```python
from build123d import *
from OCP.BRepFilletAPI import BRepFilletAPI_MakeChamfer

# Parameters (mm, degrees)
SKETCH1_W           = 60.325
SKETCH1_H           = 60.325
SKETCH1_R           = 1.778
SKETCH1_R_2         = 1.524
BOSS_EXTRUDE1_DEPTH = 6
CUT_EXTRUDE1_DEPTH  = 44.076128105
FILLET7_R           = 1.27
FILLET8_R           = 1.27
FILLET9_R           = 2.54
FILLET15_R          = 5.08
SKETCH4_W           = 2.54
SKETCH4_H           = 1.5875
BOSS_EXTRUDE2_DEPTH = 6
SKETCH6_W           = 12.7
SKETCH6_H           = 6.35
BOSS_EXTRUDE3_DEPTH = 6
FILLET10_R          = 2.54
FILLET11_R          = 2.54
BOSS_EXTRUDE4_DEPTH = 6
FILLET12_R          = 5.08
FILLET13_R          = 5.08
CUT_EXTRUDE2_REACH  = 52.712
SKETCH9_W           = 6.858
SKETCH9_H           = 2.9972
CHAMFER1_SIZE       = 0.381
CHAMFER1_SIZE2      = 1.046788897
FILLET14_R          = 0.508


with BuildPart() as part:
    # Sketch1 → Boss-Extrude1 (new body)
    with BuildSketch(Plane.XY):
        Rectangle(SKETCH1_W, SKETCH1_H)
        with Locations((26.289, 23.5585)):
            Circle(SKETCH1_R, mode=Mode.SUBTRACT)
        with Locations(Location((26.289, -23.5585, 0), (0, 0, 180))):
            Circle(SKETCH1_R, mode=Mode.SUBTRACT)
        with Locations((-25.4, 25.4)):
            Circle(SKETCH1_R, mode=Mode.SUBTRACT)
        with Locations((-25.4, -25.4)):
            Circle(SKETCH1_R, mode=Mode.SUBTRACT)
        with Locations((0, 25.4)):
            Circle(SKETCH1_R_2, mode=Mode.SUBTRACT)
        Circle(SKETCH1_R_2, mode=Mode.SUBTRACT)
        with Locations((0, -25.4)):
            Circle(SKETCH1_R_2, mode=Mode.SUBTRACT)
        with Locations((-25.4, 0)):
            Circle(SKETCH1_R, mode=Mode.SUBTRACT)
        with Locations((9.95934, 0)):
            Circle(SKETCH1_R_2, mode=Mode.SUBTRACT)
        with Locations((25.4, 0)):
            Circle(SKETCH1_R, mode=Mode.SUBTRACT)
    extrude(amount=BOSS_EXTRUDE1_DEPTH)

    # Sketch5 → Cut-Extrude1 (cut, through all)
    with BuildSketch(Plane.XY.offset(6)):
        with BuildLine():
            Line((20.4978, 23.5585), (20.4978, 6.6675))
            Line((20.4978, 6.6675), (25.0825, 6.6675))
            Line((25.0825, 6.6675), (25.0825, 19.465413928))
            ThreePointArc((25.0825, 19.465413928), (22.065552787, 24.167999366), (26.289, 27.8257))
            Line((26.289, 27.8257), (30.1625, 27.8257))
            Line((30.1625, 27.8257), (30.1625, 28.5877))
            Line((30.1625, 28.5877), (23.417563983, 28.5877))
            ThreePointArc((23.417563983, 28.5877), (21.28065408, 26.46615689), (20.4978, 23.5585))
        make_face()
    cut_extrude1 = extrude(amount=-CUT_EXTRUDE1_DEPTH, mode=Mode.SUBTRACT)

    # Fillet7
    fillet7_edges = [part.edges().sort_by_distance(p)[0] for p in [
        (30.1625, 27.8257, 3),
        (25.0825, 19.465413928, 3),
        (25.0825, 6.6675, 3),
        (20.4978, 6.6675, 3),
        (30.1625, 30.1625, 3),
    ]]
    fillet(fillet7_edges, radius=FILLET7_R)

    # Mirror1: Cut-Extrude1 across plane
    add(cut_extrude1.mirror(Plane.ZX), mode=Mode.SUBTRACT)

    # Fillet8
    fillet8_edges = [part.edges().sort_by_distance(p)[0] for p in [
        (20.4978, -6.6675, 3),
        (25.0825, -6.6675, 3),
        (25.0825, -19.465413928, 3),
        (30.1625, -27.8257, 3),
        (30.1625, -30.1625, 3),
    ]]
    fillet(fillet8_edges, radius=FILLET8_R)

    # Fillet9
    fillet9_edges = [part.edges().sort_by_distance(p)[0] for p in [
        (-30.1625, 30.1625, 3),
        (-30.1625, -30.1625, 3),
    ]]
    fillet(fillet9_edges, radius=FILLET9_R)

    # Fillet15
    fillet15_edges = [part.edges().sort_by_distance(p)[0] for p in [
        (23.417563983, -28.5877, 3),
        (23.417563983, 28.5877, 3),
    ]]
    fillet(fillet15_edges, radius=FILLET15_R)

    # Sketch4 → Boss-Extrude2 (add)
    with BuildSketch(Plane.XY.offset(6)):
        with Locations((20.58162, 30.95625)):
            Rectangle(SKETCH4_W, SKETCH4_H)
        with Locations((20.58162, -30.95625)):
            Rectangle(SKETCH4_W, SKETCH4_H)
        with Locations((-20.58162, 30.95625)):
            Rectangle(SKETCH4_W, SKETCH4_H)
        with Locations((-20.58162, -30.95625)):
            Rectangle(SKETCH4_W, SKETCH4_H)
    extrude(amount=-BOSS_EXTRUDE2_DEPTH)

    # Sketch6 → Boss-Extrude3 (add)
    with BuildSketch(Plane.XY.offset(6)):
        with Locations((0, 33.3375)):
            Rectangle(SKETCH6_W, SKETCH6_H)
    boss_extrude3 = extrude(amount=-BOSS_EXTRUDE3_DEPTH)

    # Fillet10
    fillet10_edges = [part.edges().sort_by_distance(p)[0] for p in [
        (6.35, 30.1625, 3),
        (6.35, 36.5125, 3),
        (-6.35, 36.5125, 3),
        (-6.35, 30.1625, 3),
    ]]
    fillet(fillet10_edges, radius=FILLET10_R)

    # Mirror2: Boss-Extrude3 across plane
    add(boss_extrude3.mirror(Plane.ZX))

    # Fillet11
    fillet11_edges = [part.edges().sort_by_distance(p)[0] for p in [
        (-6.35, -36.5125, 3),
        (-6.35, -30.1625, 3),
        (6.35, -30.1625, 3),
        (6.35, -36.5125, 3),
    ]]
    fillet(fillet11_edges, radius=FILLET11_R)

    # Sketch7 → Boss-Extrude4 (add)
    with BuildSketch(Plane.XY.offset(6)):
        Polygon((-21.85162, 30.1625), (21.85162, 30.1625), (21.85162, 36.5125), (21.85162, 40.3225), (10.42162, 40.3225), (10.42162, 36.5125), (-10.42162, 36.5125), (-10.42162, 40.3225), (-21.85162, 40.3225), (-21.85162, 36.5125), align=None)
        Polygon((-21.85162, -30.1625), (21.85162, -30.1625), (21.85162, -36.5125), (21.85162, -40.3225), (10.42162, -40.3225), (10.42162, -36.5125), (-10.42162, -36.5125), (-10.42162, -40.3225), (-21.85162, -40.3225), (-21.85162, -36.5125), align=None)
    extrude(amount=-BOSS_EXTRUDE4_DEPTH)

    # Fillet12
    # the kernel refuses this fillet: 5.08 mm, written as the material it takes off along each edge
    with BuildSketch(Plane(origin=(-10.42162, -40.3225, 18.296722124), x_dir=(0, 1, 0), z_dir=(0, 0, -1)), Plane(origin=(10.42162, 40.3225, 18.296722124), x_dir=(0, -1, 0), z_dir=(0, 0, -1))) as fillet12_piece_1:
        with BuildLine():
            CenterArc((5.08, -4.91868885), FILLET12_R, 104.477512186, 75.522487814)
            Line((0, -4.91868885), (-0.1016, -4.91868885))
            Line((-0.1016, -4.91868885), (-0.1016, 0))
            Line((-0.1016, 0), (0, 0.1016))
            ThreePointArc((0, 0.1016), (1.905, 0.1016), (3.7846, 0.098373777))
            Line((3.7846, 0.098373777), (3.81, 0))
        make_face()
    extrude(amount=30.593444248, mode=Mode.SUBTRACT)
    with BuildSketch(Plane(origin=(10.42162, -40.3225, 18.296722124), x_dir=(1, 0, 0), z_dir=(0, 0, -1)), Plane(origin=(-10.42162, 40.3225, 18.296722124), x_dir=(-1, 0, 0), z_dir=(0, 0, -1))) as fillet12_piece_2:
        with BuildLine():
            CenterArc((4.91868885, -5.08), FILLET12_R, 90, 75.522487814)
            Line((0, -3.81), (-0.098373777, -3.7846))
            ThreePointArc((-0.098373777, -3.7846), (-0.1016, -1.905), (-0.1016, 0))
            Line((-0.1016, 0), (0, 0.1016))
            Line((0, 0.1016), (4.91868885, 0.1016))
            Line((4.91868885, 0.1016), (4.91868885, 0))
        make_face()
    extrude(amount=30.593444248, mode=Mode.SUBTRACT)

    # Fillet13
    fillet13_edges = [part.edges().sort_by_distance(p)[0] for p in [
        (10.42162, 36.5125, 3),
        (-10.42162, 36.5125, 3),
        (-10.42162, -36.5125, 3),
        (10.42162, -36.5125, 3),
    ]]
    fillet(fillet13_edges, radius=FILLET13_R)

    # Sketch9 → Cut-Extrude2 (cut, up to next)
    with BuildSketch(Plane(origin=(0, 0, 0), x_dir=(-1, 0, 0), z_dir=(0, 0, -1)), mode=Mode.PRIVATE) as cut_extrude2_sk1:
        with Locations((-18.42262, 34.2265)):
            Rectangle(SKETCH9_W, SKETCH9_H)
    cut_extrude2_tool1 = extrude(cut_extrude2_sk1.sketch, amount=-CUT_EXTRUDE2_REACH, mode=Mode.PRIVATE) & part.part
    # Sketch9 → Cut-Extrude2 (cut, up to next)
    with BuildSketch(Plane(origin=(0, 0, 0), x_dir=(-1, 0, 0), z_dir=(0, 0, -1)), mode=Mode.PRIVATE) as cut_extrude2_sk2:
        with Locations((18.42262, 34.2265)):
            Rectangle(SKETCH9_W, SKETCH9_H)
    cut_extrude2_tool2 = extrude(cut_extrude2_sk2.sketch, amount=-CUT_EXTRUDE2_REACH, mode=Mode.PRIVATE) & part.part
    # Sketch9 → Cut-Extrude2 (cut, up to next)
    with BuildSketch(Plane(origin=(0, 0, 0), x_dir=(-1, 0, 0), z_dir=(0, 0, -1)), mode=Mode.PRIVATE) as cut_extrude2_sk3:
        with Locations((-18.42262, -34.2265)):
            Rectangle(SKETCH9_W, SKETCH9_H)
    cut_extrude2_tool3 = extrude(cut_extrude2_sk3.sketch, amount=-CUT_EXTRUDE2_REACH, mode=Mode.PRIVATE) & part.part
    # Sketch9 → Cut-Extrude2 (cut, up to next)
    with BuildSketch(Plane(origin=(0, 0, 0), x_dir=(-1, 0, 0), z_dir=(0, 0, -1)), mode=Mode.PRIVATE) as cut_extrude2_sk4:
        with Locations((18.42262, -34.2265)):
            Rectangle(SKETCH9_W, SKETCH9_H)
    cut_extrude2_tool4 = extrude(cut_extrude2_sk4.sketch, amount=-CUT_EXTRUDE2_REACH, mode=Mode.PRIVATE) & part.part
    add(cut_extrude2_tool1.solids().sort_by_distance((18.42262, 34.2265, 0))[0], mode=Mode.SUBTRACT)
    add(cut_extrude2_tool2.solids().sort_by_distance((-18.42262, 34.2265, 0))[0], mode=Mode.SUBTRACT)
    add(cut_extrude2_tool3.solids().sort_by_distance((18.42262, -34.2265, 0))[0], mode=Mode.SUBTRACT)
    add(cut_extrude2_tool4.solids().sort_by_distance((-18.42262, -34.2265, 0))[0], mode=Mode.SUBTRACT)

    # Chamfer1: one chamfer whose edges measure the first distance from different faces: ONE call of the kernel's chamfer builder (chamfer() names one face for all edges)
    chamfer1_edges_1 = [part.edges().sort_by_distance(p)[0] for p in [
        (21.85162, 32.7279, 3),
    ]]
    chamfer1_side_1 = [part.faces().sort_by_distance(p)[0] for p in [
        (21.85162, 31.4452, 3),
    ]]
    chamfer1_edges_2 = [part.edges().sort_by_distance(p)[0] for p in [
        (21.85162, 35.7251, 3),
    ]]
    chamfer1_side_2 = [part.faces().sort_by_distance(p)[0] for p in [
        (21.85162, 38.0238, 3),
    ]]
    chamfer1_edges_3 = [part.edges().sort_by_distance(p)[0] for p in [
        (-21.85162, 35.7251, 3),
    ]]
    chamfer1_side_3 = [part.faces().sort_by_distance(p)[0] for p in [
        (-21.85162, 38.0238, 3),
    ]]
    chamfer1_edges_4 = [part.edges().sort_by_distance(p)[0] for p in [
        (-21.85162, 32.7279, 3),
    ]]
    chamfer1_side_4 = [part.faces().sort_by_distance(p)[0] for p in [
        (-21.85162, 31.4452, 3),
    ]]
    chamfer1_edges_5 = [part.edges().sort_by_distance(p)[0] for p in [
        (21.85162, -35.7251, 3),
    ]]
    chamfer1_side_5 = [part.faces().sort_by_distance(p)[0] for p in [
        (21.85162, -38.0238, 3),
    ]]
    chamfer1_edges_6 = [part.edges().sort_by_distance(p)[0] for p in [
        (21.85162, -32.7279, 3),
    ]]
    chamfer1_side_6 = [part.faces().sort_by_distance(p)[0] for p in [
        (21.85162, -31.4452, 3),
    ]]
    chamfer1_edges_7 = [part.edges().sort_by_distance(p)[0] for p in [
        (-21.85162, -32.7279, 3),
    ]]
    chamfer1_side_7 = [part.faces().sort_by_distance(p)[0] for p in [
        (-21.85162, -31.4452, 3),
    ]]
    chamfer1_edges_8 = [part.edges().sort_by_distance(p)[0] for p in [
        (-21.85162, -35.7251, 3),
    ]]
    chamfer1_side_8 = [part.faces().sort_by_distance(p)[0] for p in [
        (-21.85162, -38.0238, 3),
    ]]
    chamfer1 = BRepFilletAPI_MakeChamfer(part.part.solid().wrapped)
    for e in chamfer1_edges_1:
        chamfer1.Add(CHAMFER1_SIZE, CHAMFER1_SIZE2, e.wrapped, chamfer1_side_1[0].wrapped)  # the first distance lies on this face
    for e in chamfer1_edges_2:
        chamfer1.Add(CHAMFER1_SIZE, CHAMFER1_SIZE2, e.wrapped, chamfer1_side_2[0].wrapped)  # the first distance lies on this face
    for e in chamfer1_edges_3:
        chamfer1.Add(CHAMFER1_SIZE, CHAMFER1_SIZE2, e.wrapped, chamfer1_side_3[0].wrapped)  # the first distance lies on this face
    for e in chamfer1_edges_4:
        chamfer1.Add(CHAMFER1_SIZE, CHAMFER1_SIZE2, e.wrapped, chamfer1_side_4[0].wrapped)  # the first distance lies on this face
    for e in chamfer1_edges_5:
        chamfer1.Add(CHAMFER1_SIZE, CHAMFER1_SIZE2, e.wrapped, chamfer1_side_5[0].wrapped)  # the first distance lies on this face
    for e in chamfer1_edges_6:
        chamfer1.Add(CHAMFER1_SIZE, CHAMFER1_SIZE2, e.wrapped, chamfer1_side_6[0].wrapped)  # the first distance lies on this face
    for e in chamfer1_edges_7:
        chamfer1.Add(CHAMFER1_SIZE, CHAMFER1_SIZE2, e.wrapped, chamfer1_side_7[0].wrapped)  # the first distance lies on this face
    for e in chamfer1_edges_8:
        chamfer1.Add(CHAMFER1_SIZE, CHAMFER1_SIZE2, e.wrapped, chamfer1_side_8[0].wrapped)  # the first distance lies on this face
    add(Compound.cast(chamfer1.Shape()), mode=Mode.REPLACE)

    # Fillet14
    fillet14_edges = [part.edges().sort_by_distance(p)[0] for p in [
        (14.99362, 35.7251, 3),
        (14.99362, 32.7279, 3),
        (-14.99362, 32.7279, 3),
        (-14.99362, 35.7251, 3),
        (14.99362, -32.7279, 3),
        (14.99362, -35.7251, 3),
        (-14.99362, -35.7251, 3),
        (-14.99362, -32.7279, 3),
    ]]
    fillet(fillet14_edges, radius=FILLET14_R)


solid = part.part
```
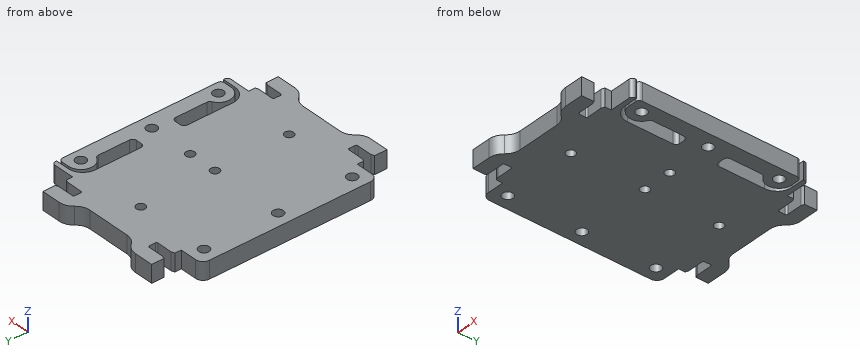
Geometry check sheet. Reference: the model listing, model coordinates, mm. Coordinates: 2 decimals unless noted, no trailing zeros. Write each loop counter-clockwise with the first axis right and the second up, starting at its lowest first coordinate (ties: lowest second). Pieces come first, ordered by that corner, then holes. Notation, with made-up numbers: M -19,-9 L 6,-9 A28 cw 6,29 Z; hole C 17,80.5 d1. An arc over 180 degrees is marked long. Answer as a JSON object with one key per item and string values.
1. Section check B-B, the plane x = -18. Enter the section's corners in (y, z).
Answers below:
{"outline": "M -40.32,0 L -35.73,0 L -35.73,6 L -40.32,6 Z; M -32.73,0 L 32.73,0 L 32.73,6 L -32.73,6 Z; M 35.73,0 L 40.32,0 L 40.32,6 L 35.73,6 Z"}
2. Go/stop test with flat-tipped pins: pin 1 Ø1 at (x, y) = (-20.5, -1.5) entering from -Z; pin 2 Ø2.5 at (x, z) = (28, 2.5) entering from +Y; pin 3 Ø3.5 at (y, z) = (-39, 4) entering from -X; pin 4 Ø1.8 at (x, z) = (-0.5, 2.5) entering from +Y. Record where each tip stops, or that it passes through.
Answers below:
{"pin 1": "stops at z = 0", "pin 2": "stops at y = 30.16", "pin 3": "stops at x = -21.85", "pin 4": "stops at y = 36.51"}
3. Scan lines: L1, parallel to Y at x = 0, z = 2; L2, parallel to Y at x = -25.4, z = 2.75; L3, parallel to Y at x = -17, z = 1.5. Record each from-to range of solid material in increasing order.
Answers below:
{"L1": "y = -36.51 to -26.92, -23.88 to -1.52, 1.52 to 23.88, 26.92 to 36.51", "L2": "y = -30.16 to -27.18, -23.62 to -1.78, 1.78 to 23.62, 27.18 to 30.16", "L3": "y = -40.32 to -35.73, -32.73 to 32.73, 35.73 to 40.32"}
4. Section check C-C, the plane x = -25.4. Enter the section's corners in (y, z), plus the area to 3 significant figures.
Answers below:
{"outline": "M -30.16,0 L -27.18,0 L -27.18,6 L -30.16,6 Z; M -23.62,0 L -1.78,0 L -1.78,6 L -23.62,6 Z; M 1.78,0 L 23.62,0 L 23.62,6 L 1.78,6 Z; M 27.18,0 L 30.16,0 L 30.16,6 L 27.18,6 Z", "area": "298 mm²"}
5. Section check A-A, the plane y = 0. Enter the section's corners in (x, z).
Answers below:
{"outline": "M -30.16,0 L -27.18,0 L -27.18,6 L -30.16,6 Z; M -23.62,0 L -1.52,0 L -1.52,6 L -23.62,6 Z; M 1.52,0 L 8.44,0 L 8.44,6 L 1.52,6 Z; M 11.48,0 L 23.62,0 L 23.62,6 L 11.48,6 Z; M 27.18,0 L 30.16,0 L 30.16,6 L 27.18,6 Z"}
6. Section check D-D, the plane y = 16. Enter the section's corners in (x, z), plus the area to 3 significant figures.
Answers below:
{"outline": "M -30.16,0 L 20.5,0 L 20.5,6 L -30.16,6 Z; M 25.08,0 L 30.16,0 L 30.16,6 L 25.08,6 Z", "area": "334 mm²"}
